Read the model definition and answer for the solid it produces. Units are mm, in the model's axes. A direction names the side the tool comes from. Coordinates: 2 decimals unless noted, no trailing zeros. Order: outer loops, then holes, each group sorted by start corner. A loop starts at its lowest first (then second) coordinate and runs counter-clockwise, first axis right, second up. Notation, with made-up numbers: M 67.5,70 L 79.5,70 A15 ccw 79.5,96 Z; hole C 60,1 d1. An arc over 180 degrees is marked long. Put each result on its own line as item: value.
from build123d import *

# Parameters (mm, degrees)
F0_W      = 6
F0_H      = 3
F1_DEPTH  = 15
F4_DEPTH  = 80
F2_W      = 2.7
F2_H      = 15.4
F5_DEPTH  = 10
F2_R      = 1.7
F6_DEPTH  = 25
F2_R_2    = 3.5
F7_DEPTH  = 25
F8_DEPTH  = 10
F9_W      = 10
F9_H      = 25
F10_DEPTH = 25
F11_R     = 1.7
F13_DEPTH = 50
F14_DEPTH = 50
F12_R     = 1.7
F15_DEPTH = 6
F16_DEPTH = 10
F17_DEPTH = 18
F18_R     = 1.7
F19_DEPTH = 6
F20_DEPTH = 25
F21_DEPTH = 18
F22_DEPTH = 80


with BuildPart() as f1:
    # F0 (on Front) → F1 (new body)
    with BuildSketch(Plane.XZ):
        with BuildLine():
            Line((35, 70), (-35, 70))
            ThreePointArc((-35, 70), (-38.5355339059, 68.5355339059), (-40, 65))
            Line((-40, 65), (-40, -65))
            ThreePointArc((-40, -65), (-38.5355339059, -68.5355339059), (-35, -70))
            Line((-35, -70), (35, -70))
            ThreePointArc((35, -70), (38.5355339059, -68.5355339059), (40, -65))
            Line((40, -65), (40, 65))
            ThreePointArc((40, 65), (38.5355339059, 68.5355339059), (35, 70))
        make_face()
        with Locations((0, -57)):
            Rectangle(F0_W, F0_H, mode=Mode.SUBTRACT)
        with Locations((0, 57)):
            Rectangle(F0_W, F0_H, mode=Mode.SUBTRACT)
    extrude(amount=F1_DEPTH)

    # F3 (on face) → F4 (cut)
    with BuildSketch(Plane(origin=(-40, 0, 0), x_dir=(0, -1, 0), z_dir=(-1, 0, 0))):
        with BuildLine():
            ThreePointArc((0, 32.3), (5.4447222151, 34.5552777849), (7.7, 40))
            ThreePointArc((7.7, 40), (5.4447222151, 45.4447222151), (0, 47.7))
            Line((0, 47.7), (0, 44.5))
            ThreePointArc((0, 44.5), (3.1819805153, 43.1819805153), (4.5, 40))
            ThreePointArc((4.5, 40), (3.1819805153, 36.8180194847), (0, 35.5))
            Line((0, 35.5), (0, 32.3))
        make_face()
        with BuildLine():
            ThreePointArc((7.7, -40), (5.4447222151, -34.5552777849), (0, -32.3))
            Line((0, -32.3), (0, -35.5))
            ThreePointArc((0, -35.5), (3.1819805153, -36.8180194847), (4.5, -40))
            ThreePointArc((4.5, -40), (3.1819805153, -43.1819805153), (0, -44.5))
            Line((0, -44.5), (0, -47.7))
            ThreePointArc((0, -47.7), (5.4447222151, -45.4447222151), (7.7, -40))
        make_face()
    extrude(amount=-F4_DEPTH, mode=Mode.SUBTRACT)

    # F2 (on face) → F5 (join)
    with BuildSketch(Plane(origin=(0, 0, 0), x_dir=(-1, 0, 0), z_dir=(0, 1, 0))):
        with Locations((-38.65, 40)):
            Rectangle(F2_W, F2_H)
        Polygon((12.7, 47.7), (0, 47.7), (-12.7, 47.7), (-12.7, 32.3), (0, 32.3), (12.7, 32.3), align=None)
        with Locations((38.65, 40)):
            Rectangle(F2_W, F2_H)
        with Locations((-38.65, -40)):
            Rectangle(F2_W, F2_H)
        Polygon((0, -32.3), (-12.7, -32.3), (-12.7, -47.7), (0, -47.7), (12.7, -47.7), (12.7, -32.3), align=None)
        with Locations((38.65, -40)):
            Rectangle(F2_W, F2_H)
    extrude(amount=-F5_DEPTH)

    # F2 (on face) → F6 (cut)
    with BuildSketch(Plane(origin=(0, 0, 0), x_dir=(-1, 0, 0), z_dir=(0, 1, 0))):
        with Locations((-25, 61.7)):
            Circle(F2_R)
        with Locations((25, 61.7)):
            Circle(F2_R)
        with Locations((-25, 18.3)):
            Circle(F2_R)
        with Locations((25, 18.3)):
            Circle(F2_R)
        with Locations((-25, -18.3)):
            Circle(F2_R)
        with Locations((25, -18.3)):
            Circle(F2_R)
        with Locations((-25, -61.7)):
            Circle(F2_R)
        with Locations((25, -61.7)):
            Circle(F2_R)
    extrude(amount=-F6_DEPTH, mode=Mode.SUBTRACT)

    # F2 (on face) → F7 (cut)
    with BuildSketch(Plane(origin=(0, 0, 0), x_dir=(-1, 0, 0), z_dir=(0, 1, 0))):
        with Locations((-25, 61.7)):
            Circle(F2_R_2)
        with Locations((-25, 61.7)):
            Circle(F2_R, mode=Mode.SUBTRACT)
        with Locations((25, 61.7)):
            Circle(F2_R_2)
        with Locations((25, 61.7)):
            Circle(F2_R, mode=Mode.SUBTRACT)
        with Locations((-25, 18.3)):
            Circle(F2_R_2)
        with Locations((-25, 18.3)):
            Circle(F2_R, mode=Mode.SUBTRACT)
        with Locations((25, 18.3)):
            Circle(F2_R_2)
        with Locations((25, 18.3)):
            Circle(F2_R, mode=Mode.SUBTRACT)
        with Locations((-25, -18.3)):
            Circle(F2_R_2)
        with Locations((-25, -18.3)):
            Circle(F2_R, mode=Mode.SUBTRACT)
        with Locations((25, -18.3)):
            Circle(F2_R_2)
        with Locations((25, -18.3)):
            Circle(F2_R, mode=Mode.SUBTRACT)
        with Locations((-25, -61.7)):
            Circle(F2_R_2)
        with Locations((-25, -61.7)):
            Circle(F2_R, mode=Mode.SUBTRACT)
        with Locations((25, -61.7)):
            Circle(F2_R_2)
        with Locations((25, -61.7)):
            Circle(F2_R, mode=Mode.SUBTRACT)
    extrude(amount=-F7_DEPTH, mode=Mode.SUBTRACT)

    # F2 (on face) → F8 (join)
    with BuildSketch(Plane(origin=(0, 0, 0), x_dir=(-1, 0, 0), z_dir=(0, 1, 0))):
        with Locations((-25, 61.7)):
            Circle(F2_R_2)
        with Locations((-25, 61.7)):
            Circle(F2_R, mode=Mode.SUBTRACT)
        with Locations((25, 61.7)):
            Circle(F2_R_2)
        with Locations((25, 61.7)):
            Circle(F2_R, mode=Mode.SUBTRACT)
        with Locations((-25, 18.3)):
            Circle(F2_R_2)
        with Locations((-25, 18.3)):
            Circle(F2_R, mode=Mode.SUBTRACT)
        with Locations((25, 18.3)):
            Circle(F2_R_2)
        with Locations((25, 18.3)):
            Circle(F2_R, mode=Mode.SUBTRACT)
        with Locations((-25, -18.3)):
            Circle(F2_R_2)
        with Locations((-25, -18.3)):
            Circle(F2_R, mode=Mode.SUBTRACT)
        with Locations((25, -18.3)):
            Circle(F2_R_2)
        with Locations((25, -18.3)):
            Circle(F2_R, mode=Mode.SUBTRACT)
        with Locations((-25, -61.7)):
            Circle(F2_R_2)
        with Locations((-25, -61.7)):
            Circle(F2_R, mode=Mode.SUBTRACT)
        with Locations((25, -61.7)):
            Circle(F2_R_2)
        with Locations((25, -61.7)):
            Circle(F2_R, mode=Mode.SUBTRACT)
    extrude(amount=-F8_DEPTH)

    # F9 (on face) → F10 (join)
    with BuildSketch(Plane.XZ.offset(15)):
        Rectangle(F9_W, F9_H)
    extrude(amount=F10_DEPTH)

    # F11 (on face) → F13 (cut, symmetric)
    with BuildSketch(Plane.YZ.offset(5)):
        with BuildLine():
            ThreePointArc((-15, -4.2473521163), (-13.3826414478, -2.3916521486), (-12.8, 0))
            ThreePointArc((-12.8, 0), (-13.3826414478, 2.3916521486), (-15, 4.2473521163))
            Line((-15, 4.2473521163), (-15, -4.2473521163))
        make_face()
        with BuildLine():
            Line((-15, -4.2473521163), (-15, 4.2473521163))
            ThreePointArc((-15, 4.2473521163), (-23.2, 0), (-15, -4.2473521163))
        make_face()
        with Locations((-18, 8)):
            Circle(F11_R)
        with Locations((-26, 0)):
            Circle(F11_R)
        with Locations((-18, -8)):
            Circle(F11_R)
        with Locations((-10, 0)):
            Circle(F11_R)
        with BuildLine():
            ThreePointArc((-18, -12.5), (-30.5, 0), (-18, 12.5))
            Line((-18, 12.5), (-40, 12.5))
            Line((-40, 12.5), (-40, -12.5))
            Line((-40, -12.5), (-18, -12.5))
        make_face()
    extrude(amount=F13_DEPTH, both=True, mode=Mode.SUBTRACT)

    # F11 (on face) → F14 (cut, symmetric)
    with BuildSketch(Plane.YZ.offset(5)):
        with BuildLine():
            ThreePointArc((-15, -4.2473521163), (-23.2, 0), (-15, 4.2473521163))
            Line((-15, 4.2473521163), (-15, 12.1346610995))
            ThreePointArc((-15, 12.1346610995), (-16.4889182259, 12.408329133), (-18, 12.5))
            ThreePointArc((-18, 12.5), (-30.5, 0), (-18, -12.5))
            ThreePointArc((-18, -12.5), (-16.4889182259, -12.408329133), (-15, -12.1346610995))
            Line((-15, -12.1346610995), (-15, -4.2473521163))
        make_face()
        with Locations((-18, -8)):
            Circle(F11_R, mode=Mode.SUBTRACT)
        with Locations((-26, 0)):
            Circle(F11_R, mode=Mode.SUBTRACT)
        with Locations((-18, 8)):
            Circle(F11_R, mode=Mode.SUBTRACT)
        with BuildLine():
            ThreePointArc((-15, 4.2473521163), (-13.3826414478, 2.3916521486), (-12.8, 0))
            ThreePointArc((-12.8, 0), (-13.3826414478, -2.3916521486), (-15, -4.2473521163))
            Line((-15, -4.2473521163), (-15, -12.1346610995))
            ThreePointArc((-15, -12.1346610995), (-8.1574901575, -7.7055175037), (-5.5, 0))
            ThreePointArc((-5.5, 0), (-8.1574901575, 7.7055175037), (-15, 12.1346610995))
            Line((-15, 12.1346610995), (-15, 4.2473521163))
        make_face()
        with Locations((-10, 0)):
            Circle(F11_R, mode=Mode.SUBTRACT)
    extrude(amount=F14_DEPTH, both=True, mode=Mode.SUBTRACT)

    # F12 (on face) → F15 (cut)
    with BuildSketch(Plane.XY.offset(70)):
        Polygon((12, 0), (0, 0), (-12, 0), (-12, -15), (12, -15), align=None)
        with Locations((0, -7.5)):
            Circle(F12_R, mode=Mode.SUBTRACT)
    extrude(amount=-F15_DEPTH, mode=Mode.SUBTRACT)

    # F11 (on face) → F16 (join)
    with BuildSketch(Plane.YZ.offset(5)):
        with BuildLine():
            ThreePointArc((-15, -4.2473521163), (-23.2, 0), (-15, 4.2473521163))
            Line((-15, 4.2473521163), (-15, 12.1346610995))
            ThreePointArc((-15, 12.1346610995), (-16.4889182259, 12.408329133), (-18, 12.5))
            ThreePointArc((-18, 12.5), (-30.5, 0), (-18, -12.5))
            ThreePointArc((-18, -12.5), (-16.4889182259, -12.408329133), (-15, -12.1346610995))
            Line((-15, -12.1346610995), (-15, -4.2473521163))
        make_face()
        with Locations((-18, -8)):
            Circle(F11_R, mode=Mode.SUBTRACT)
        with Locations((-26, 0)):
            Circle(F11_R, mode=Mode.SUBTRACT)
        with Locations((-18, 8)):
            Circle(F11_R, mode=Mode.SUBTRACT)
        with BuildLine():
            ThreePointArc((-15, 4.2473521163), (-13.3826414478, 2.3916521486), (-12.8, 0))
            ThreePointArc((-12.8, 0), (-13.3826414478, -2.3916521486), (-15, -4.2473521163))
            Line((-15, -4.2473521163), (-15, -12.1346610995))
            ThreePointArc((-15, -12.1346610995), (-8.1574901575, -7.7055175037), (-5.5, 0))
            ThreePointArc((-5.5, 0), (-8.1574901575, 7.7055175037), (-15, 12.1346610995))
            Line((-15, 12.1346610995), (-15, 4.2473521163))
        make_face()
        with Locations((-10, 0)):
            Circle(F11_R, mode=Mode.SUBTRACT)
    extrude(amount=-F16_DEPTH)

    # F12 (on face) → F17 (cut)
    with BuildSketch(Plane.XY.offset(70)):
        with Locations((0, -7.5)):
            Circle(F12_R)
    extrude(amount=-F17_DEPTH, mode=Mode.SUBTRACT)

    # F18 (on face) → F19 (cut)
    with BuildSketch(Plane(origin=(0, 0, -70), x_dir=(1, 0, 0), z_dir=(0, 0, -1))):
        Polygon((-12, 0), (0, 0), (12, 0), (12, 15), (-12, 15), align=None)
        with Locations((0, 7.5)):
            Circle(F18_R, mode=Mode.SUBTRACT)
    extrude(amount=-F19_DEPTH, mode=Mode.SUBTRACT)

    # F0 (on Front) → F20 (cut)
    with BuildSketch(Plane.XZ):
        with Locations((0, -57)):
            Rectangle(F0_W, F0_H)
    extrude(amount=-F20_DEPTH, mode=Mode.SUBTRACT)

    # F18 (on face) → F21 (cut)
    with BuildSketch(Plane(origin=(0, 0, -70), x_dir=(1, 0, 0), z_dir=(0, 0, -1))):
        with Locations((0, 7.5)):
            Circle(F18_R)
    extrude(amount=-F21_DEPTH, mode=Mode.SUBTRACT)

    # F3 (on face) → F22 (cut)
    with BuildSketch(Plane(origin=(-40, 0, 0), x_dir=(0, -1, 0), z_dir=(-1, 0, 0))):
        with BuildLine():
            ThreePointArc((4.5, -40), (3.1819805153, -36.8180194847), (0, -35.5))
            Line((0, -35.5), (0, -44.5))
            ThreePointArc((0, -44.5), (3.1819805153, -43.1819805153), (4.5, -40))
        make_face()
        with BuildLine():
            Line((0, -44.5), (0, -35.5))
            ThreePointArc((0, -35.5), (-4.5, -40), (0, -44.5))
        make_face()
        with BuildLine():
            Line((0, 35.5), (0, 44.5))
            ThreePointArc((0, 44.5), (-4.5, 40), (0, 35.5))
        make_face()
        with BuildLine():
            ThreePointArc((4.5, 40), (3.1819805153, 43.1819805153), (0, 44.5))
            Line((0, 44.5), (0, 35.5))
            ThreePointArc((0, 35.5), (3.1819805153, 36.8180194847), (4.5, 40))
        make_face()
    extrude(amount=-F22_DEPTH, mode=Mode.SUBTRACT)


solid = f1.part
Q1. Find section A-A on z = 61.7. Write down the section's boundary in (x, y), plus the area to 3 significant figures.
Answers below:
outline: M -40,-15 L -28.5,-15 L -28.5,-10 L -26.7,-10 L -26.7,0 L -40,0 Z; M -23.3,-10 L -21.5,-10 L -21.5,-15 L 21.5,-15 L 21.5,-10 L 23.3,-10 L 23.3,0 L -23.3,0 Z; M 26.7,-10 L 28.5,-10 L 28.5,-15 L 40,-15 L 40,0 L 26.7,0 Z; hole C 0,-7.5 d3.4
area: 1,050 mm^2
Q2. Find section B-B on x = -32. Write down the section's boundary in (y, z), plus the area to 3 significant figures.
Answers below:
outline: M -15,-70 L 0,-70 L 0,-47.7 A7.7 cw 0,-32.3 L 0,32.3 A7.7 cw 0,47.7 L 0,70 L -15,70 L -15,12.13 A12.5 cw -15,-12.13 Z
area: 1,740 mm^2
Q3. For a pull along Z with two mould halves and no side action, classify faces 4 (the face through (-12, -8, -67)), 5 (the face through (37.3, -5, 40)), 6 (the face through (-0.7, -5.7, -55.5)), 7 (the face through (0, -16, 12.5)) as +Z half, -Z half, draft (parallel to the pull), parting line (faces both ways), or undercut.
Answers below:
face 4: draft
face 5: undercut
face 6: undercut
face 7: +Z half
Q4. Consider line 1 along Z through (x, y) = (-2.5, -18); line 2 along Z through (x, y) = (-21.5, -4); line 3 along Z through (x, y) = (-25, -12). Determine where each line is inside the solid, lowest interval first.
Answers below:
line 1: z = -12.5 to -9.7, -6.3 to -5.2, 5.2 to 6.3, 9.7 to 12.5
line 2: z = -70 to -46.58, -33.42 to 33.42, 46.58 to 70
line 3: z = -70 to -65.2, -58.2 to -21.8, -14.8 to -10.97, 10.97 to 14.8, 21.8 to 58.2, 65.2 to 70
Q5. A tool of negligible diameter and unlimited length cuts with its end or side. For faces 1 (the face through (-12, -7, 67)), 2 (the face through (-27, -10, 19)), 3 (the face through (2, -8, -64)), from which of +Z, -Z, +X, -X, +Y, -Y can it reach the whole face along a straight path? Write none if from no direction.
Answers below:
face 1: +Z, +Y, -Y
face 2: -Y
face 3: -Z, +Y, -Y
Q6. Given pin 1 (3.5 mm diameter, centred on x = -2, y = -16.5, fed in from -Z); pin 2 (7.5 mm diameter, centred on x = -24.5, z = 19, fed in from -Y); pin 3 (6 mm diameter, centred on x = -0.5, y = -16.5, fed in from +Z); pin 4 (2 mm diameter, centred on x = 25, z = 61.7, fed in from +Y), each flat-ended and moving along its own axis, determine where each tip first touches the part or whether it passes through.
Answers below:
pin 1: stops at z = -64
pin 2: stops at y = -15
pin 3: stops at z = 64
pin 4: passes through
Q7. Find section D-D on y = -26. Write down the section's boundary in (x, z), plus the area to 3 significant figures.
Answers below:
outline: M -5,-9.6 L 5,-9.6 L 5,-1.7 L -5,-1.7 Z; M -5,1.7 L 5,1.7 L 5,9.6 L -5,9.6 Z
area: 158 mm^2
Q8. Find section C-C on x = 0. Give the number of separate pieces and of enclosed holes in the cut face, plus the area to 3 significant figures.
Answers below:
separate pieces: 5
enclosed holes: 5
area: 1,900 mm^2
